from build123d import *

# Parameters (mm, degrees)
F0_W     = 107.95
F0_H     = 60.325
F0_W_2   = 85.725
F0_H_2   = 41.275
F1_DEPTH = 1.5875
F2_DEPTH = 11.1125
F3_R     = 2.032


with BuildPart() as f1:
    # F0 (on Front) → F1 (new body)
    with BuildSketch(Plane.XZ):
        with Locations((1.5875, 0)):
            Rectangle(F0_W, F0_H)
        Rectangle(F0_W_2, F0_H_2, mode=Mode.SUBTRACT)
        Rectangle(F0_W_2, F0_H_2)
    extrude(amount=F1_DEPTH)

    # F0 (on Front) → F2 (join)
    with BuildSketch(Plane.XZ):
        Rectangle(F0_W_2, F0_H_2)
    extrude(amount=F2_DEPTH)

    # F3
    f3_edges = [f1.edges().sort_by_distance(p)[0] for p in [
        (42.8625, -6.35, 20.6375),
        (-42.8625, -6.35, 20.6375),
        (-42.8625, -6.35, -20.6375),
        (42.8625, -6.35, -20.6375),
        (42.8625, -11.1125, 0),
        (0, -11.1125, -20.6375),
        (-42.8625, -11.1125, 0),
        (0, -11.1125, 20.6375),
    ]]
    fillet(f3_edges, radius=F3_R)


solid = f1.part
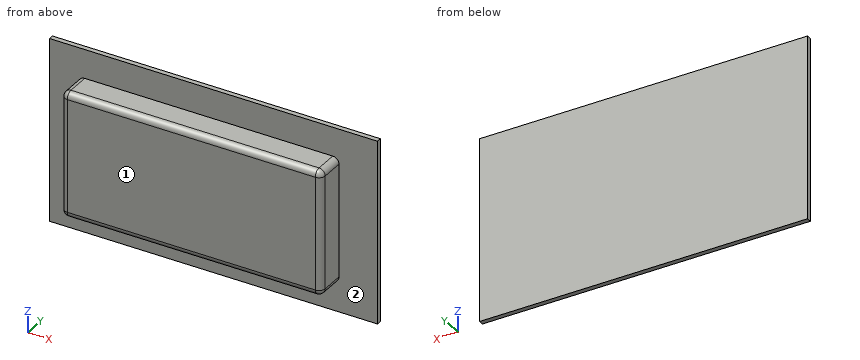
Can you work these out from the model? Positions are in its coordinate system, mm. Face numbers are marked on the shaded views. A direction names the side the tool comes from. Round coordinates to 2 decimals unless told otherwise and drop trailing zeros. Order: outer loops, then holes, each group sorted by start corner. A loop starts at its lowest first (then second) coordinate and runs counter-clockwise, first axis right, second up. Notation, with made-up numbers: (-5, 70.25) -> (31, 70.25) arc R18 cw to (31, 94.25) -> close; hole circle Ø1 at (74, 76.25). An arc over 180 degrees is marked (long way). Write each question's results on one line, items separated by ' | '. Start each with the question number.
Item 1: If we section it at D-D, the plane x = -46: Write out the boundary of the cut face in (y, z), then the cut area to 3 significant figures.
Item 2: If we section it at C-C, the plane z = -15.5: Write out the boundary of the cut face in (x, y), then the cut area to 3 significant figures.
Item 3: If we section it at A-A, the plane y = -6.75: Write out the boundary of the cut face in (x, z), then the cut area to 3 significant figures.
Item 4: If we section it at B-B, the plane x = 17: Write out the boundary of the cut face in (y, z), then the cut area to 3 significant figures.
Item 5: Which directions (+Z, -Z, +X, -X, +Y, -Y) give clear straight access to the entire face, cutting with the end or side of a thin tool? Please do the marked faces 1 and 2.
Item 6: Please list where these lines run through material, in increasing order: L1, parallel to Z at x = -34, y = -3; L2, parallel to Y at x = 27.5, z = -25; L3, parallel to X at y = -1.75, z = 17.5.
Item 7: Will these pins go through, and if not, where does the flat tip stop? pin 1 (3.5 mm diameter, centred on x = 17, y = -6, fed in from +Z); pin 2 (2 mm diameter, centred on y = -6.5, z = -8, fed in from -X); pin 3 (3.5 mm diameter, centred on y = -4.5, z = 6, fed in from +X).
Results:
1) outline: (-1.59, -30.16) -> (0, -30.16) -> (0, 30.16) -> (-1.59, 30.16) -> close | area: 95.8 mm2
2) outline: (-52.39, -1.59) -> (-42.86, -1.59) -> (-42.86, -9.08) arc R2.03 ccw to (-40.83, -11.11) -> (40.83, -11.11) arc R2.03 ccw to (42.86, -9.08) -> (42.86, -1.59) -> (55.56, -1.59) -> (55.56, 0) -> (-52.39, 0) -> close | area: 986 mm2
3) outline: (-42.86, -18.61) arc R2.03 ccw to (-40.83, -20.64) -> (40.83, -20.64) arc R2.03 ccw to (42.86, -18.61) -> (42.86, 18.61) arc R2.03 ccw to (40.83, 20.64) -> (-40.83, 20.64) arc R2.03 ccw to (-42.86, 18.61) -> close | area: 3,530 mm2
4) outline: (-11.11, -18.61) arc R2.03 ccw to (-9.08, -20.64) -> (-1.59, -20.64) -> (-1.59, -30.16) -> (0, -30.16) -> (0, 30.16) -> (-1.59, 30.16) -> (-1.59, 20.64) -> (-9.08, 20.64) arc R2.03 ccw to (-11.11, 18.61) -> close | area: 487 mm2
5) face 1: +Z, -Z, +X, -X, -Y | face 2: -Y
6) L1: z = -20.64 to 20.64 | L2: y = -1.59 to 0 | L3: x = -42.86 to 42.86
7) pin 1: stops at z = 20.64 | pin 2: stops at x = -42.86 | pin 3: stops at x = 42.86
